Autodesk Inventor part; units mm, degrees
ref_plane "YZ Plane" through (0, 0, 0) normal (1, 0, 0) x (0, 1, 0)
ref_plane "XZ Plane" through (0, 0, 0) normal (0, 1, 0) x (-1, 0, 0)
ref_plane "XY Plane" through (0, 0, 0) normal (0, 0, 1) x (1, 0, 0)
sketch "Sketch3" plane through (0, 0, 0) normal (0, 0, 1) x (1, 0, 0)
  line L0 (-13.9172, 10.4459) -> (46.0828, 10.4459)
  line L1 (46.0828, 10.4459) -> (46.0828, -4.5541)
  line L2 (46.0828, -4.5541) -> (-13.9172, -4.5541)
  line L3 (-13.9172, -4.5541) -> (-13.9172, 10.4459)
  line L4 (46.0828, -4.5541) -> (61.0828, -4.5541)
  line L5 (61.0828, -4.5541) -> (61.0828, 10.4459)
  line L6 (61.0828, 10.4459) -> (46.0828, 10.4459)
  line L7 (46.0828, 10.4459) -> (46.0828, -4.5541)
  line L8 (-13.9172, 10.4459) -> (-28.9172, 10.4459)
  line L9 (-28.9172, 10.4459) -> (-28.9172, -4.5541)
  line L10 (-28.9172, -4.5541) -> (-13.9172, -4.5541)
  line L11 (-13.9172, -4.5541) -> (-13.9172, 10.4459)
  point P0 (0, 0)
  dimension "d0" = 15
  dimension "d1" = 15
  dimension "d2" = 15
  dimension "d3" = 60
extrude "Extrusion1" add sketch "Sketch3" along normal blind 10 contours L0 L1 L2 L3
extrude "Extrusion2" add sketch "Sketch3" along normal blind 40 contours L3 L10 L9 L8 | L6 L5 L4 L1
equation "\"d2\" = d1"
properties part number "HandleR01"
Model file for the job. Use its own axes, mm. A direction names the side the tool comes from. Give positions to 0.01 mm unless a question says otherwise; leave off trailing zeros. Write each loop counter-clockwise with the first axis right and the second up, starting at its lowest first coordinate (ties: lowest second). Pieces come first, ordered by that corner, then holes. Notation, with made-up numbers: (59.25, 20.25) - (116.25, 20.25) arc R9 cw to (116.25, 25.25) - close; hole circle Ø11 at (24, -38.5). An arc over 180 degrees is marked (long way). Answer as CSV lines item,"result".
1. Band-saw the part on C-C (x = 28.5). Write the cut outline in (y, z).
Responses:
outline,"(-4.55, 0) - (10.45, 0) - (10.45, 10) - (-4.55, 10) - close"
2. 3-axis set-ups, long thin cutter, end or side, ignore diameter. For faces 1 (the face through (46.083, 3, 25)), 2 (the face through (27, -4.554, 6)): which of +Z, -Z, +X, -X, +Y, -Y reach the whole face in a straight line?
Responses:
face 1,"+Z, +Y, -Y"
face 2,"+Z, -Z, +X, -X, -Y"
3. Band-saw the part on B-B (y = 3.5). Write the cut outline in (x, z).
Responses:
outline,"(-28.92, 0) - (61.08, 0) - (61.08, 40) - (46.08, 40) - (46.08, 10) - (-13.92, 10) - (-13.92, 40) - (-28.92, 40) - close"
4. Band-saw the part on A-A (z = 36). Write the cut outline in (x, y).
Responses:
outline,"(-28.92, -4.55) - (-13.92, -4.55) - (-13.92, 10.45) - (-28.92, 10.45) - close; (46.08, -4.55) - (61.08, -4.55) - (61.08, 10.45) - (46.08, 10.45) - close"
5. Drill centre lines: L1, parallel to X at y = -2.5, z = 30.5; L2, parallel to Z at x = 26, y = -3.5. Where is each one in solid material? Low to high. Write a range as [from, to].
Responses:
L1,"x = [-28.92, -13.92], [46.08, 61.08]"
L2,"z = [0, 10]"
6. Pin check, flat tip, straight feed: pin 1 (4.5 mm diameter, centred on x = 16.5, y = 1, fed in from +Z). Stop position of the tip, or through.
Responses:
pin 1,"stops at z = 10"
7. Two-plate mould, pull along X, no slides. Class faces 3 (the face through (-13.917, 3, 25)), 4 (the face through (16, 3, 10)), 5 (the face through (-28.917, 3, 20)), 6 (the face through (15, 3, 0)): +X half, -X half, draft (parallel to the pull), parting line (faces both ways), or undercut.
Responses:
face 3,"undercut"
face 4,"undercut"
face 5,"-X half"
face 6,"draft"
